Source: CAD feature listing. Evaluate the final solid. Frame: model axes, mm. A direction names the side the tool comes from. Give positions to 0.01 mm unless a question says otherwise; leave off trailing zeros. Order: outer loops, then holes, each group sorted by start corner. A loop starts at its lowest first (then second) coordinate and runs counter-clockwise, first axis right, second up.
1) Access query for faces 1 (the face through (12.5, -2.24, -0.05)), 2 (the face through (-0.05, -2.24, -12.5)), 3 (the face through (12.5, 2.24, -0.05)), 4 (the face through (-0.05, 2.24, -12.5)). Directions: +Z, -Z, +X, -X, +Y, -Y. A direction counts if a zero-diameter tool reaches every point of the face in a straight line with its end or side. Return the directions, or none.
2) First-contact query: P1, Ø2.5, axis at y = 0, z = 16.9, coming from the -X side; P2, Ø1.5, axis at y = 0, z = 9.5, coming from the -X side; P3, Ø3.5, axis at y = 0, z = -16.9, coming from the +X side; P4, Ø3, axis at y = 1, z = -16, coming from the -X side. Flat tips, straight axial feed; report the tip coordinate or a pass-through.
3) Material intervals for line 1 (X direction, y = -0.5, z = -4); line 2 (X direction, y = 0.5, z = 14.5); line 3 (Z direction, x = 8, y = 0.25), sorted ascending.
4) Section D-D, the plane y = 0.75. Give the number of separate pieces and of enclosed holes in the cut face, plus the area to 3 significant figures.
5) Section B-B, the plane z = 0. Return loops of the section in (x, y), plus the area to 3 significant figures.
6) Draft query along X for faces 5 (the face through (-18.33, 0.45, 6.36)), 6 (the face through (-10.833, -2.593, 10.77)), 7 (the face through (15, 0, 8.9)). Return one class per face: released by +X, released by -X, zero draft, split by the parting line, or undercut.
7) Section A-A, the plane x = 0. Return loops of the section in (y, z).
8) Section C-C, the plane x = -14. Return loops of the section in (y, z), plus the area to 3 significant figures.
```python
from build123d import *

# Parameters (mm, degrees)
SKETCH1_R           = 2.5
BOSS_EXTRUDE1_DEPTH = 3.1
SKETCH2_R           = 1.5
CUT_EXTRUDE1_DEPTH  = 36.836573497
CIRPATTERN1_COUNT   = 4
FILLET1_R           = 3
CHAMFER1_SIZE       = 1
CHAMFER3_SIZE       = 0.5


with BuildPart() as part:
    # Sketch1 → Boss-Extrude1 (new, symmetric)
    with BuildSketch(Plane(origin=(0, 0, 0), x_dir=(1, 0, 0), z_dir=(0, 1, 0))):
        Polygon((-8.9, -13.4), (-8.9, -20.4), (-3.9, -20.4), (-3.9, -13.4), (3.9, -13.4), (3.9, -20.4), (8.9, -20.4), (8.9, -13.4), (13.4, -8.9), (20.4, -8.9), (20.4, -3.9), (13.4, -3.9), (13.4, 3.9), (20.4, 3.9), (20.4, 8.9), (13.4, 8.9), (8.9, 13.4), (8.9, 20.4), (3.9, 20.4), (3.9, 13.4), (-3.9, 13.4), (-3.9, 20.4), (-8.9, 20.4), (-8.9, 13.4), (-13.4, 8.9), (-20.4, 8.9), (-20.4, 3.9), (-13.4, 3.9), (-13.4, -3.9), (-20.4, -3.9), (-20.4, -8.9), (-13.4, -8.9), align=None)
        with Locations(Location((0, 0, 0), (0, 0, 90))):
            Circle(SKETCH1_R, mode=Mode.SUBTRACT)
    extrude(amount=BOSS_EXTRUDE1_DEPTH, both=True)

    # Sketch2 → Cut-Extrude1 (cut, symmetric)
    with BuildSketch(Plane.ZY.offset(8.9)):
        with Locations((16.9, 0)):
            Circle(SKETCH2_R)
        with BuildLine():
            Line((16.9, 3.1), (20.4, 3.1))
            Line((20.4, 3.1), (20.4, -3.1))
            Line((20.4, -3.1), (16.9, -3.1))
            ThreePointArc((16.9, -3.1), (20, 0), (16.9, 3.1))
        make_face()
    cut_extrude1 = extrude(amount=CUT_EXTRUDE1_DEPTH, both=True, mode=Mode.SUBTRACT)

    # CirPattern1: Cut-Extrude1 ×4 about axis
    cirpattern1_axis = Axis((0, 3.1, 0), (0, 1, 0))
    for i in range(1, CIRPATTERN1_COUNT):
        add(cut_extrude1.rotate(cirpattern1_axis, i * 360 / CIRPATTERN1_COUNT), mode=Mode.SUBTRACT)

    # Fillet1
    fillet1_edges = [part.edges().sort_by_distance(p)[0] for p in [
        (-13.4, 3.1, 0),
        (0, 3.1, 13.4),
        (-13.4, -3.1, 0),
        (0, -3.1, -13.4),
        (13.4, -3.1, 0),
        (0, -3.1, 13.4),
        (13.4, 3.1, 0),
        (0, 3.1, -13.4),
    ]]
    fillet(fillet1_edges, radius=FILLET1_R)

    # Chamfer1
    chamfer1_edges = [part.edges().sort_by_distance(p)[0] for p in [
        (-11.15, 3.1, -11.15),
        (-11.15, -3.1, -11.15),
        (11.15, -3.1, -11.15),
        (11.15, 3.1, 11.15),
        (11.15, -3.1, 11.15),
        (-11.15, -3.1, 11.15),
        (-11.15, 3.1, 11.15),
        (11.15, 3.1, -11.15),
    ]]
    chamfer(chamfer1_edges, length=CHAMFER1_SIZE)

    # Chamfer3
    chamfer3_edges = [part.edges().sort_by_distance(p)[0] for p in [
        (0, -3.1, 2.5),
        (0, 3.1, 2.5),
    ]]
    chamfer(chamfer3_edges, length=CHAMFER3_SIZE)


solid = part.part
```
From the geometry:
1. face 1: +X, -Y
1. face 2: -Z, -Y
1. face 3: +X, +Y
1. face 4: -Z, +Y
2. P1: passes through
2. P2: stops at x = -20
2. P3: stops at x = 8.9
2. P4: stops at x = -8.9
3. line 1: x = -19.96 to -18.31, -15.49 to 15.49, 18.31 to 19.96
3. line 2: x = -8.9 to -3.9, 3.9 to 8.9
3. line 3: z = -19.99 to -18.38, -15.42 to 15.42, 18.38 to 19.99
4. separate pieces: 9
4. enclosed holes: 1
4. area: 812 mm2
5. outline: (-13.4, -0.1) arc R3 ccw to (-10.4, -3.1) - (-3, -3.1) - (-2.5, -2.6) - (-2.5, 2.6) - (-3, 3.1) - (-10.4, 3.1) arc R3 ccw to (-13.4, 0.1) - close; (2.5, -2.6) - (3, -3.1) - (10.4, -3.1) arc R3 ccw to (13.4, -0.1) - (13.4, 0.1) arc R3 ccw to (10.4, 3.1) - (3, 3.1) - (2.5, 2.6) - close
5. area: 127 mm2
6. face 5: undercut
6. face 6: released by -X
6. face 7: zero draft
7. outline: (-3.1, -10.4) arc R3 ccw to (-0.1, -13.4) - (0.1, -13.4) arc R3 ccw to (3.1, -10.4) - (3.1, -3) - (2.6, -2.5) - (-2.6, -2.5) - (-3.1, -3) - close; (-3.1, 3) - (-2.6, 2.5) - (2.6, 2.5) - (3.1, 3) - (3.1, 10.4) arc R3 ccw to (0.1, 13.4) - (-0.1, 13.4) arc R3 ccw to (-3.1, 10.4) - close
8. outline: (-3.1, -8.9) - (3.1, -8.9) - (3.1, -3.9) - (-3.1, -3.9) - close; (-3.1, 3.9) - (3.1, 3.9) - (3.1, 8.9) - (-3.1, 8.9) - close
8. area: 62.0 mm2
